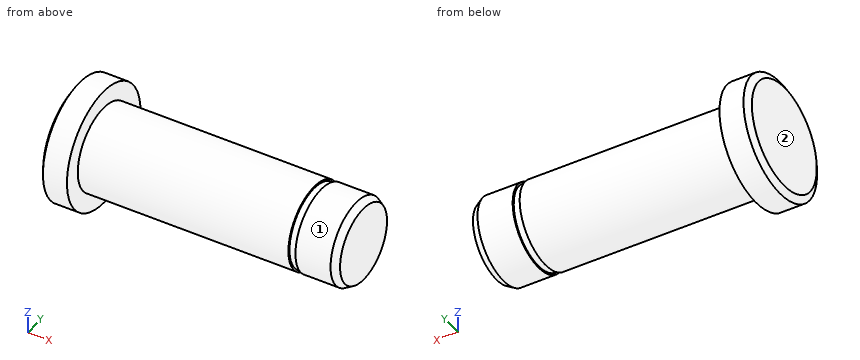
from build123d import *

# Parameters (mm, degrees)
SFAZOWANIE1_SIZE           = 1
SFAZOWANIE1_SIZE2          = 0.577350269
SFAZOWANIE1_PART_2_SIZE    = 1
SFAZOWANIE1_PART_2_SIZE2   = 0.577350269
WYTNIJ_WYCI_GNI_CIE1_START = -6
SZKIC2_R                   = 6
SZKIC2_R_2                 = 5.75
WYTNIJ_WYCI_GNI_CIE1_DEPTH = 1


with BuildPart() as part:
    # Szkic1 → Obrót1 (revolve)
    with BuildSketch(Plane.XY):
        Polygon((0, 0), (0, 8.5), (4, 8.5), (4, 6), (41, 6), (41, 0), align=None)
    revolve(axis=Axis((41, 0, 0), (-1, 0, 0)))

    # Sfazowanie1
    sfazowanie1_edges = [part.edges().sort_by_distance(p)[0] for p in [
        (41, -6, 0),
    ]]
    sfazowanie1_side = [part.faces().sort_by_distance(p)[0] for p in [
        (22.5, -6, 0),
    ]]
    chamfer(sfazowanie1_edges, length=SFAZOWANIE1_SIZE, length2=SFAZOWANIE1_SIZE2, reference=sfazowanie1_side[0])

    # Sfazowanie1 part 2
    sfazowanie1_part_2_edges = [part.edges().sort_by_distance(p)[0] for p in [
        (0, -8.5, 0),
    ]]
    sfazowanie1_part_2_side = [part.faces().sort_by_distance(p)[0] for p in [
        (0, 0, 0),
    ]]
    chamfer(sfazowanie1_part_2_edges, length=SFAZOWANIE1_PART_2_SIZE, length2=SFAZOWANIE1_PART_2_SIZE2, reference=sfazowanie1_part_2_side[0])

    # Szkic2 → Wytnij-wyciągnięcie1 (cut)
    with BuildSketch(Plane(origin=(41, 0, 0), x_dir=(0, 0, -1), z_dir=(1, 0, 0)).offset(WYTNIJ_WYCI_GNI_CIE1_START)):
        Circle(SZKIC2_R)
        Circle(SZKIC2_R_2, mode=Mode.SUBTRACT)
    extrude(amount=-WYTNIJ_WYCI_GNI_CIE1_DEPTH, mode=Mode.SUBTRACT)


solid = part.part
CAD build for the part. Positions are in the model's coordinates, mm. Face numbers are marked on the shaded views. A direction names the side the tool comes from. Give positions to 0.01 mm unless a question says otherwise; leave off trailing zeros. Order: outer loops, then holes, each group sorted by start corner. A loop starts at its lowest first (then second) coordinate and runs counter-clockwise, first axis right, second up. Notation, with made-up numbers: (30, 15) - (62, 15) arc R24 ccw to (62, 48) - close; hole circle Ø8 at (-16, 7.5). An arc over 180 degrees is marked (long way). Write each question's results on one line, items separated by ' | '.
1. Probe L1, parallel to X at y = 6.75, z = 3; L2, parallel to X at y = 5.75, z = 1.5; L3, parallel to Y at x = 2.5, z = 0.5. List the from-to ranges inside material, lowest first. Write a range as from..to.
Calculated:
L1: x = 0..4 | L2: x = 0..34, 35..40.1 | L3: y = -8.49..8.49
2. Pin check, flat tips, straight feed: pin 1 (1.5 mm diameter, centred on y = 3.5, z = -2.5, fed in from -X); pin 2 (1.5 mm diameter, centred on x = 4.5, z = -4, fed in from +Y); pin 3 (6 mm diameter, centred on x = 26, y = -3.5, fed in from +Z); pin 4 (1 mm diameter, centred on y = 3, z = -5.5, fed in from +X). Stop position of each tip, or through.
Calculated:
pin 1: stops at x = 0 | pin 2: stops at y = 7.77 | pin 3: stops at z = 5.98 | pin 4: stops at x = 40.41
3. 3-axis set-ups, long thin cutter, end or side, ignore diameter. For the marked faces 1 and 2: which of +Z, -Z, +X, -X, +Y, -Y reach the whole face in a straight line?
Calculated:
face 1: +X | face 2: +Z, -Z, -X, +Y, -Y
4. Saw through at C-C on x = 12. List the corners of the cut face in (y, z), and give its area (3 significant figures).
Calculated:
outline: circle Ø12 at (0, 0) | area: 113 mm2
5. Saw through at A-A on y = 0. List the corners of the cut face in (x, z), and give its area (3 significant figures).
Calculated:
outline: (0, -7.5) - (0.58, -8.5) - (4, -8.5) - (4, -6) - (34, -6) - (34, -5.75) - (35, -5.75) - (35, -6) - (40, -6) - (41, -5.42) - (41, 5.42) - (40, 6) - (35, 6) - (35, 5.75) - (34, 5.75) - (34, 6) - (4, 6) - (4, 8.5) - (0.58, 8.5) - (0, 7.5) - close | area: 510 mm2
